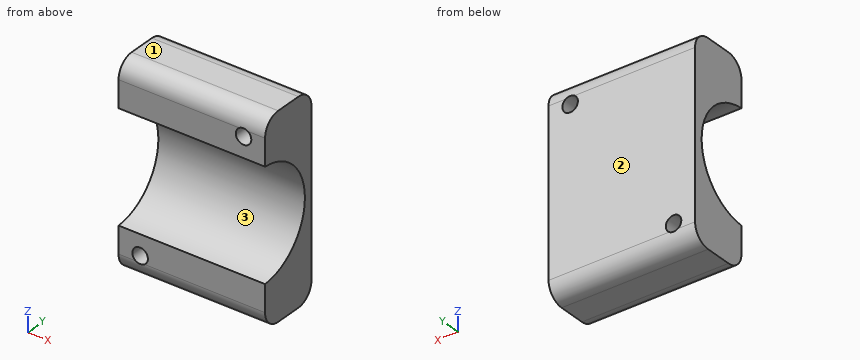
```python
from build123d import *

# Parameters (mm, degrees)
BOSS_EXTRUDE1_DEPTH     = 17
CUT_EXTRUDE1_DEPTH      = 33.20310544
CUT_EXTRUDE1_DEPTH_BACK = 33.20310544
SKETCH2_R               = 12.8
SKETCH3_R               = 1.8
CUT_EXTRUDE2_DEPTH      = 14.8


with BuildPart() as part:
    # Sketch1 → Boss-Extrude1 (new, symmetric)
    with BuildSketch(Plane(origin=(0, 0, 0), x_dir=(0, 0, -1), z_dir=(1, 0, 0))):
        with BuildLine():
            Line((-19, 0.6), (19, 0.6))
            ThreePointArc((19, 0.6), (21.828427125, 1.771572875), (23, 4.6))
            Line((23, 4.6), (23, 10.8))
            ThreePointArc((23, 10.8), (21.828427125, 13.628427125), (19, 14.8))
            Line((19, 14.8), (-19, 14.8))
            ThreePointArc((-19, 14.8), (-21.828427125, 13.628427125), (-23, 10.8))
            Line((-23, 10.8), (-23, 4.6))
            ThreePointArc((-23, 4.6), (-21.828427125, 1.771572875), (-19, 0.6))
        make_face()
    extrude(amount=BOSS_EXTRUDE1_DEPTH, both=True)

    # Sketch2 → Cut-Extrude1 (cut, two sides: drawn at the far end of the back side and taken through both)
    with BuildSketch(Plane(origin=(0, 0, 0), x_dir=(0, 0, -1), z_dir=(1, 0, 0)).offset(-CUT_EXTRUDE1_DEPTH_BACK)):
        Circle(SKETCH2_R)
    extrude(amount=CUT_EXTRUDE1_DEPTH + CUT_EXTRUDE1_DEPTH_BACK, mode=Mode.SUBTRACT)

    # Sketch3 → Cut-Extrude2 (cut)
    with BuildSketch(Plane(origin=(0, 0.6, 0), x_dir=(1, 0, 0), z_dir=(0, 1, 0))):
        with Locations(Location((12, -17.5, 0), (0, 0, 236.442690238))):
            Circle(SKETCH3_R)
        with Locations(Location((-12, 17.5, 0), (0, 0, 123.557309762))):
            Circle(SKETCH3_R)
    extrude(amount=CUT_EXTRUDE2_DEPTH, mode=Mode.SUBTRACT)


solid = part.part
```
Can you work these out from the model? Positions are in its coordinate system, mm. Face numbers are marked on the shaded views. Coordinates: 2 decimals unless noted, no trailing zeros. Loops run counter-clockwise (first coordinate to the right, second up) from the corner with the lowest first, then second, coordinate; pieces in that order, holes last.
1) Thinking about a two-plate mould opening in Z: for the marked faces 1, 2 and 3, which applies, pulls with the +Z half, pulls with the -Z half, needs draft (parallel to the pull), parting line crosses it, or undercut?
2) Imagine slicing it at B-B on z = 17.5. List the corners of the cut face in (x, y) for me, plus the area to 3 significant figures.
3) Imagine slicing it at C-C on x = 12. List the corners of the cut face in (y, z) for me.
4) Imagine slicing it at D-D on x = -8.5. List the corners of the cut face in (y, z) for me, plus the area to 3 significant figures.
5) For pin 1 (3 mm diameter, centred on x = 12, z = 17.5, fed in from -Y), with a flat end and sliding along its axis, tell me the tip position at first contact or that it passes through.
6) Imagine slicing it at A-A on y = 6. List the corners of the cut face in (x, z) for me, plus the area to 3 significant figures.
7) I need wall thicknesses on probe 1 along X at (y, z) = (5.5, 17.5); probe 2 along Z at (x, y) = (13, 9.5); probe 3 along Z at (x, y) = (-12, 11.75). Which ranges of each line are inside material? Lowest first, please.
Completed:
1. face 1: pulls with the +Z half
1. face 2: needs draft
1. face 3: undercut
2. outline: (-17, 0.6) - (10.2, 0.6) - (10.2, 14.8) - (-17, 14.8) - close; (13.8, 0.6) - (17, 0.6) - (17, 14.8) - (13.8, 14.8) - close
2. area: 432 mm2
3. outline: (0.6, -19) arc R4 ccw to (4.6, -23) - (10.8, -23) arc R4 ccw to (14.8, -19) - (14.8, 15.7) - (0.6, 15.7) - (0.6, 12.79) arc R12.8 cw to (0.6, -12.79) - close; (0.61, 19.3) - (14.79, 19.3) arc R4 ccw to (10.8, 23) - (4.6, 23) arc R4 ccw to start
4. outline: (0.6, -19) arc R4 ccw to (4.6, -23) - (10.8, -23) arc R4 ccw to (14.8, -19) - (14.8, 19) arc R4 ccw to (10.8, 23) - (4.6, 23) arc R4 ccw to (0.6, 19) - (0.6, 12.79) arc R12.8 cw to (0.6, -12.79) - close
4. area: 397 mm2
5. pin 1: passes through
6. outline: (-17, -23) - (17, -23) - (17, -11.31) - (-17, -11.31) - close; (-17, 11.31) - (17, 11.31) - (17, 23) - (-17, 23) - close; hole circle Ø3.6 at (-12, -17.5); hole circle Ø3.6 at (12, 17.5)
6. area: 775 mm2
7. probe 1: x = -17 to 10.2, 13.8 to 17
7. probe 2: z = -23 to -8.58, 8.58 to 16, 19 to 23
7. probe 3: z = -22.89 to -19.3, -15.7 to -5.08, 5.08 to 22.89
